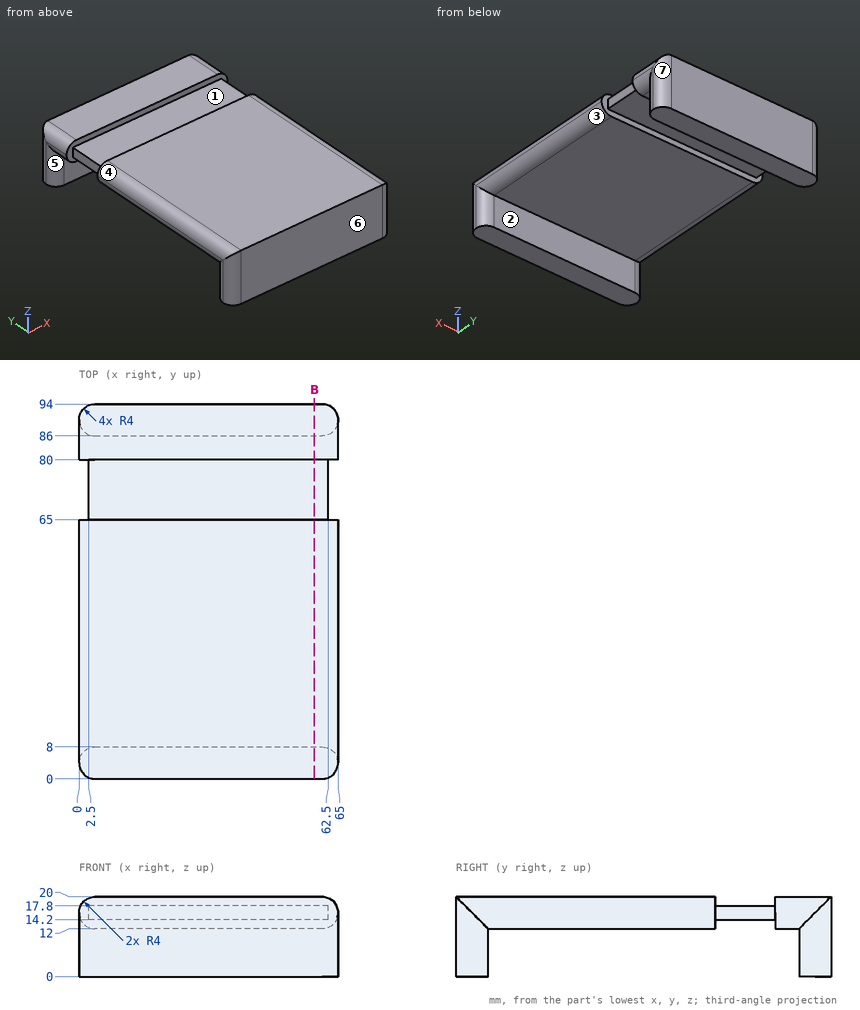
Answer from the drawing. Dimensions are ordinates in mm from the lowest x, y and z of the part. A direction names the side the tool comes from. Round coordinates to 2 decimals unless told otherwise and drop trailing zeros. Loops run counter-clockwise (first coordinate to the right, second up) from the corner with the lowest first, then second, coordinate; pieces in that order, holes last.
(1) Each of these flat-tipped pins is pushed along its axis until it touches: P1, Ø8, axis at x = 39, y = 41, coming from the -Z side; P2, Ø3, axis at y = 72.5, z = 15.5, coming from the -X side; P3, Ø1.1, axis at y = 70.5, z = 15.5, coming from the +X side. Where does it stop, or does it pass through?
Computed values:
P1: stops at z = 12
P2: stops at x = 2.5
P3: stops at x = 62.5
(2) The mould has two halves that part along Y. Classify the marked faces 4, 5, 6 and 7: pulls with the +Y half, pulls with the -Y half, needs draft (parallel to the pull), parting line crosses it, or undercut.
Computed values:
face 4: needs draft
face 5: undercut
face 6: pulls with the -Y half
face 7: pulls with the +Y half
(3) For the marked faces 1, 2 and 3, determine the directions among +Z, -Z, +X, -X, +Y, -Y from which every point of the face is accessible in a straight line to the end or side of a thin tool.
Computed values:
face 1: +Z, +X, -X
face 2: -Z, +X, -X
face 3: -Z, +X
(4) The part is cut by section B-B, the plane x = 59. Give the vertices of the cut face in (y, z).
Computed values:
outline: (0, 0) - (8, 0) - (8, 12) - (65, 12) - (65, 14.2) - (80, 14.2) - (80, 12) - (86, 12) - (86, 0) - (94, 0) - (94, 20) - (80, 20) - (80, 17.8) - (65, 17.8) - (65, 20) - (0, 20) - close
(5) Find the intervals of material crossed by L1, parallel to Y at x = 23, z = 1.75; L2, parallel to Y at x = 11.5, z = 19.25; L3, parallel to Z at x = 60.5, y = 22, in increasing order.
Computed values:
L1: y = 0 to 8, 86 to 94
L2: y = 0 to 65, 80 to 94
L3: z = 12 to 20
